Part model, mm, in its own coordinate system. Face numbers are marked on the shaded views. A direction names the side the tool comes from. Round coordinates to 2 decimals unless told otherwise and drop trailing zeros. Loops run counter-clockwise (first coordinate to the right, second up) from the corner with the lowest first, then second, coordinate; pieces in that order, holes last. Notation, with made-up numbers: (-15.5, 79) -> (2.5, 79) arc R27 ccw to (2.5, 105) -> close; hole circle Ø6 at (77, 15). An arc over 180 degrees is marked (long way). Use a Markdown table: item, result. Add a question column.
Item 1: Which spindle directions (+Z, -Z, +X, -X, +Y, -Y) get a long thin tool onto all of the face, cutting with end or side? Do the marked faces 4 and 5. Say none if no direction does.
Item 2: Cut at D-D, the plane x = 1. List the corners of the cut face in (y, z).
Item 3: Probe line 1 (X direction, y = 0.75, z = -8.5); line 2 (Z direction, x = 14, y = 0.65); line 3 (X direction, y = 4.05, z = 6.5). List the from-to ranges inside material, lowest first. Write a range as [from, to].
Item 4: Cut at A-A, the plane z = 7.5. List the corners of the cut face in (x, y).
Item 5: Cut at B-B, the plane x = 12. List the corners of the cut face in (y, z), plus the area to 3 significant figures.
Item 6: Cut at C-C, the plane z = 2. List the corners of the cut face in (x, y), plus the area to 3 significant figures.
Item 7: Two-plate mould, pull along Z, no slides. Class the marked faces 1, 2 and 3: pulls with the +Z half, pulls with the -Z half, needs draft (parallel to the pull), parting line crosses it, or undercut.
```python
from build123d import *

# Parameters (mm, degrees)
SKETCH1_W           = 36.81984
SKETCH1_H           = 36.81984
SKETCH1_W_2         = 3.81
SKETCH1_H_2         = 5.08
SKETCH1_W_3         = 5.08
SKETCH1_H_3         = 3.81
BOSS_EXTRUDE1_DEPTH = 5.08


with BuildPart() as part:
    # Sketch1 → Boss-Extrude1 (new body)
    with BuildSketch(Plane(origin=(0, 0, 0), x_dir=(1, 0, 0), z_dir=(0, 1, 0))):
        with Locations((0.909996046, -2.939987224)):
            Rectangle(SKETCH1_W, SKETCH1_H)
        Polygon((0.909996046, 4.680012776), (3.449996046, 4.680012776), (3.449996046, -0.399987224), (8.529996046, -0.399987224), (8.529996046, -2.939987224), (8.529996046, -5.479987224), (3.449996046, -5.479987224), (3.449996046, -10.559987224), (0.909996046, -10.559987224), (-1.630003954, -10.559987224), (-1.630003954, -5.479987224), (-6.710003954, -5.479987224), (-6.710003954, -2.939987224), (-6.710003954, -0.399987224), (-1.630003954, -0.399987224), (-1.630003954, 4.680012776), align=None, mode=Mode.SUBTRACT)
        with Locations((5.354996046, 7.849932776)):
            Rectangle(SKETCH1_W_2, SKETCH1_H_2, mode=Mode.SUBTRACT)
        with Locations((-3.535003954, 7.849932776)):
            Rectangle(SKETCH1_W_2, SKETCH1_H_2, mode=Mode.SUBTRACT)
        with Locations((11.699916046, -7.384987224)):
            Rectangle(SKETCH1_W_3, SKETCH1_H_3, mode=Mode.SUBTRACT)
        with Locations((11.699916046, 1.505012776)):
            Rectangle(SKETCH1_W_3, SKETCH1_H_3, mode=Mode.SUBTRACT)
        with Locations((-3.535003954, -13.729907224)):
            Rectangle(SKETCH1_W_2, SKETCH1_H_2, mode=Mode.SUBTRACT)
        with Locations((5.354996046, -13.729907224)):
            Rectangle(SKETCH1_W_2, SKETCH1_H_2, mode=Mode.SUBTRACT)
        with Locations((-9.879923954, 1.505012776)):
            Rectangle(SKETCH1_W_3, SKETCH1_H_3, mode=Mode.SUBTRACT)
        with Locations((-9.879923954, -7.384987224)):
            Rectangle(SKETCH1_W_3, SKETCH1_H_3, mode=Mode.SUBTRACT)
    extrude(amount=BOSS_EXTRUDE1_DEPTH)


solid = part.part
```
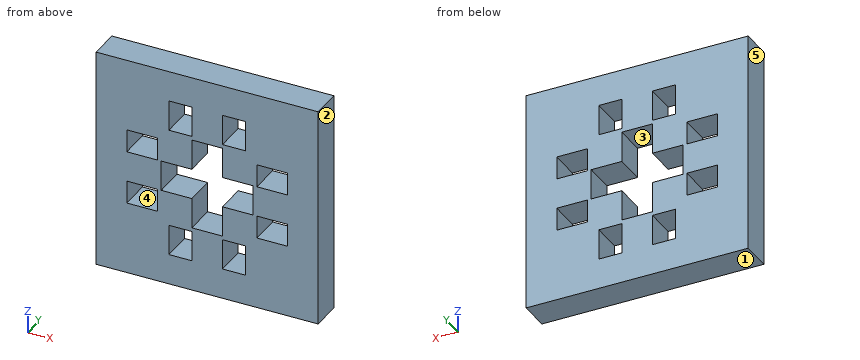
A:
| question | item | result |
|---|---|---|
| 1 | face 4 | +Y, -Y |
| 1 | face 5 | +Z, -Z, -X, +Y, -Y |
| 2 | outline | (0, -15.47) -> (5.08, -15.47) -> (5.08, -4.68) -> (0, -4.68) -> close; (0, 10.56) -> (5.08, 10.56) -> (5.08, 21.35) -> (0, 21.35) -> close |
| 3 | line 1 | x = [-17.5, -5.44], [-1.63, 3.45], [7.26, 19.32] |
| 3 | line 2 | z = [-15.47, -3.41], [0.4, 5.48], [9.29, 21.35] |
| 3 | line 3 | x = [-17.5, -12.42], [-7.34, -1.63], [3.45, 9.16], [14.24, 19.32] |
| 4 | outline | (-17.5, 0) -> (-12.42, 0) -> (-12.42, 5.08) -> (-17.5, 5.08) -> close; (-7.34, 0) -> (-1.63, 0) -> (-1.63, 5.08) -> (-7.34, 5.08) -> close; (3.45, 0) -> (9.16, 0) -> (9.16, 5.08) -> (3.45, 5.08) -> close; (14.24, 0) -> (19.32, 0) -> (19.32, 5.08) -> (14.24, 5.08) -> close |
| 5 | outline | (0, -15.47) -> (5.08, -15.47) -> (5.08, -3.41) -> (0, -3.41) -> close; (0, 0.4) -> (5.08, 0.4) -> (5.08, 5.48) -> (0, 5.48) -> close; (0, 9.29) -> (5.08, 9.29) -> (5.08, 21.35) -> (0, 21.35) -> close |
| 5 | area | 148 mm^2 |
| 6 | outline | (-17.5, 0) -> (-6.71, 0) -> (-6.71, 5.08) -> (-17.5, 5.08) -> close; (8.53, 0) -> (19.32, 0) -> (19.32, 5.08) -> (8.53, 5.08) -> close |
| 6 | area | 110 mm^2 |
| 7 | face 1 | pulls with the -Z half |
| 7 | face 2 | needs draft |
| 7 | face 3 | undercut |
